```python
from build123d import *

# Parameters (mm, degrees)
ESQUISSE1_R          = 3
BASE_EXTRUSION_DEPTH = 4
CONG_1_R             = 3
CONG_2_R             = 2


with BuildPart() as part:
    # Esquisse1 → Base-Extrusion (new body)
    with BuildSketch(Plane.XY):
        with BuildLine():
            Line((15.795884765, -7), (72.892937741, -7))
            Line((72.892937741, -7), (87.900637518, 10.264383688))
            ThreePointArc((87.900637518, 10.264383688), (97.070633478, 10.905612271), (97.711862061, 1.735616312))
            Line((97.711862061, 1.735616312), (78.817379063, -20))
            Line((78.817379063, -20), (10.277712155, -20))
            Line((10.277712155, -20), (-4.675708702, -4.515279408))
            ThreePointArc((-4.675708702, -4.515279408), (-4.515279408, 4.675708702), (4.675708702, 4.515279408))
            Line((4.675708702, 4.515279408), (15.795884765, -7))
        make_face()
        Circle(ESQUISSE1_R, mode=Mode.SUBTRACT)
        with Locations((92.80624979, 6)):
            Circle(ESQUISSE1_R, mode=Mode.SUBTRACT)
    extrude(amount=BASE_EXTRUSION_DEPTH)

    # Congé1
    cong_1_edges = [part.edges().sort_by_distance(p)[0] for p in [
        (78.817379063, -20, 2),
        (10.277712155, -20, 2),
    ]]
    fillet(cong_1_edges, radius=CONG_1_R)

    # Congé2
    cong_2_edges = [part.edges().sort_by_distance(p)[0] for p in [
        (72.892937741, -7, 2),
        (15.795884765, -7, 2),
    ]]
    fillet(cong_2_edges, radius=CONG_2_R)


solid = part.part
```
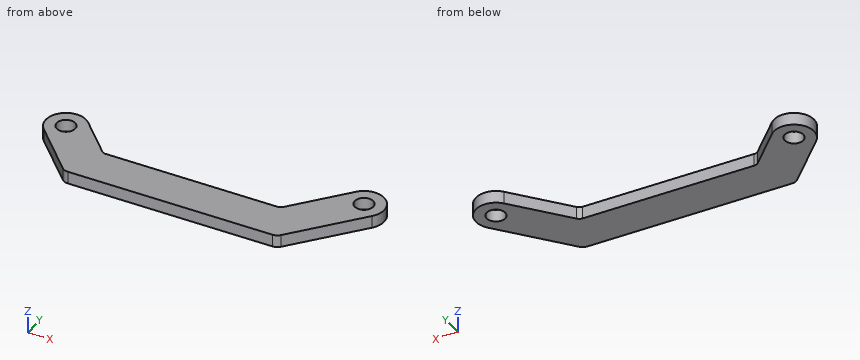
Can you work these out from the model? Positions are in its coordinate system, mm. Give positions to 0.01 mm unless a question says otherwise; leave off trailing zeros. Write each loop counter-clockwise with the first axis right and the second up, starting at its lowest first coordinate (ties: lowest second). Pieces come first, ordered by that corner, then holes. Notation, with made-up numbers: (26.25, 17.25) - (42.25, 17.25) arc R14 ccw to (42.25, 25.25) - close; hole circle Ø1 at (-34.75, -30.75). An arc over 180 degrees is marked (long way). Write item = value, one per line. Start each with the question number.
1. Imagine slicing it at B-B (z = 1.85). Please give me the cut outline in (x, y), and give its area (3 significant figures).
2. Please list where these lines run through material, in increasing order: line 1 (Y direction, x = 69, z = 0.6); line 2 (X direction, y = 2, z = 3.05); line 3 (Y direction, x = 0, z = 2.35).
3. For pin 1 (1 mm diameter, centred on y = -14, z = 3, fed in from +X); pin 2 (1.5 mm diameter, centred on y = 2, z = 2.5, fed in from +X); pin 3 (1.2 mm diameter, centred on x = 41, z = 1.5, fed in from +Y), each with a flat end and sliding along its axis, tell me the tip position at first contact or that it passes through.
4. Imagine slicing it at C-C (x = 0). Please give me the cut outline in (y, z), and give its area (3 significant figures).
5. Imagine slicing it at A-A (y = 0). Please give me the cut outline in (x, z), and give its area (3 significant figures).
6. Imagine slicing it at D-D (x = 42). Please give me the cut outline in (y, z).
Worked answers:
q1.outline = (-4.68, -4.52) - (9.39, -19.08) arc R3 ccw to (11.55, -20) - (77.45, -20) arc R3 ccw to (79.71, -18.97) - (97.71, 1.74) arc R6.5 ccw to (87.9, 10.26) - (73.49, -6.31) arc R2 cw to (71.98, -7) - (16.64, -7) arc R2 cw to (15.21, -6.39) - (4.68, 4.52) arc R6.5 ccw to start; hole circle Ø6 at (0, 0); hole circle Ø6 at (92.81, 6)
q1.area = 1,470 mm2
q2.line_1 = -20 to -7
q2.line_2 = -6.18 to -2.24, 2.24 to 7.1, 80.72 to 97.93
q2.line_3 = -9.36 to -3, 3 to 6.5
q3.pin_1 = 84.47
q3.pin_2 = 98.44
q3.pin_3 = -7
q4.outline = (-9.36, 0) - (-3, 0) - (-3, 4) - (-9.36, 4) - close; (3, 0) - (6.5, 0) - (6.5, 4) - (3, 4) - close
q4.area = 39.4 mm2
q5.outline = (-6.5, 0) - (-3, 0) - (-3, 4) - (-6.5, 4) - close; (3, 0) - (9.04, 0) - (9.04, 4) - (3, 4) - close; (78.98, 0) - (96.2, 0) - (96.2, 4) - (78.98, 4) - close
q5.area = 107 mm2
q6.outline = (-20, 0) - (-7, 0) - (-7, 4) - (-20, 4) - close
